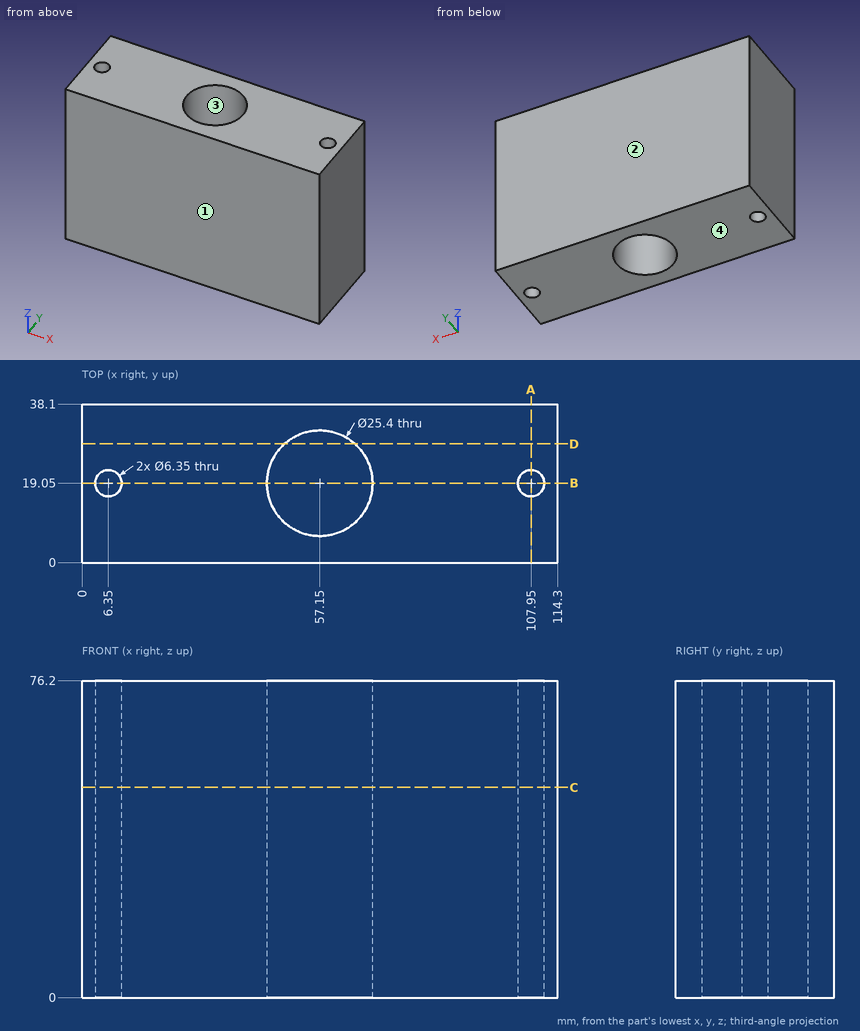
Print and shaded views of the part. All mm, measured from the part's lowest x, y and z. Give positions to 0.01 mm unless a question says otherwise; leave off trailing zeros. Loops run counter-clockwise (first coordinate to the right, second up) from the corner with the lowest first, then second, coordinate; pieces in that order, holes last. Notation, with made-up numbers: (76.5, 37) -> (107.5, 37) arc R25 cw to (107.5, 63) -> close; hole circle Ø8 at (-21, 3.5). An arc over 180 degrees is marked (long way). Use a Markdown table: item, result.
1. Flat gauge pins, fed straight in: pin 1 (10 mm diameter, centred on x = 107.95, y = 19.05, fed in from -Z); pin 2 (4 mm diameter, centred on x = 6.35, y = 19.05, fed in from +Z). Where does each tip first touch, or does it go through?
Check result:
| item | result |
|---|---|
| pin 1 | stops at z = 0 |
| pin 2 | passes through |
2. Wall check: L1, parallel to X at y = 19, z = 19; L2, parallel to Y at x = 107.95, z = 56.5 (3 decimals); L3, parallel to Y at x = 57, z = 59. Give the ranges that are in metal, low to high. Write a range as [from, to].
Check result:
| item | result |
|---|---|
| L1 | x = [0, 3.18], [9.52, 44.45], [69.85, 104.78], [111.12, 114.3] |
| L2 | y = [0, 15.875], [22.225, 38.1] |
| L3 | y = [0, 6.35], [31.75, 38.1] |
3. Mould opens along Y. For the marked faces 1, 2, 3 and 4 say: pulls with the +Y half, pulls with the -Y half, needs draft (parallel to the pull), parting line crosses it, or undercut.
Check result:
| item | result |
|---|---|
| face 1 | pulls with the -Y half |
| face 2 | pulls with the +Y half |
| face 3 | undercut |
| face 4 | needs draft |
4. Slice it at A-A (x = 107.95). List the corners of the cut face in (y, z) (3 decimals).
Check result:
| item | result |
|---|---|
| outline | (0, 0) -> (15.875, 0) -> (15.875, 76.2) -> (0, 76.2) -> close; (22.225, 0) -> (38.1, 0) -> (38.1, 76.2) -> (22.225, 76.2) -> close |
5. Slice it at C-C (z = 50.5). List the corners of the cut face in (x, y) (3 decimals), plus the area to 3 significant figures.
Check result:
| item | result |
|---|---|
| outline | (0, 0) -> (114.3, 0) -> (114.3, 38.1) -> (0, 38.1) -> close; hole circle Ø6.35 at (6.35, 19.05); hole circle Ø25.4 at (57.15, 19.05); hole circle Ø6.35 at (107.95, 19.05) |
| area | 3,780 mm^2 |
6. Slice it at D-D (y = 28.5). List the corners of the cut face in (x, z), plus the area to 3 significant figures.
Check result:
| item | result |
|---|---|
| outline | (0, 0) -> (48.67, 0) -> (48.67, 76.2) -> (0, 76.2) -> close; (65.63, 0) -> (114.3, 0) -> (114.3, 76.2) -> (65.63, 76.2) -> close |
| area | 7,420 mm^2 |
7. Slice it at B-B (y = 19.05). List the corners of the cut face in (x, z) (3 decimals), plus the area to 3 significant figures.
Check result:
| item | result |
|---|---|
| outline | (0, 0) -> (3.175, 0) -> (3.175, 76.2) -> (0, 76.2) -> close; (9.525, 0) -> (44.45, 0) -> (44.45, 76.2) -> (9.525, 76.2) -> close; (69.85, 0) -> (104.775, 0) -> (104.775, 76.2) -> (69.85, 76.2) -> close; (111.125, 0) -> (114.3, 0) -> (114.3, 76.2) -> (111.125, 76.2) -> close |
| area | 5,810 mm^2 |
